```python
from build123d import *

# Parameters (mm, degrees)
SKETCH1_R           = 6.2992
BOSS_EXTRUDE1_DEPTH = 6.477
SKETCH2_R           = 9.4615
BOSS_EXTRUDE2_DEPTH = 6.223
SKETCH5_R           = 9.4615
SKETCH6_R           = 3.3782
SKETCH7_R           = 3.0226
CUT_EXTRUDE1_DEPTH  = 31.932950796


with BuildPart() as part:
    # Sketch1 → Boss-Extrude1 (new body)
    with BuildSketch(Plane(origin=(0, 0, 0), x_dir=(1, 0, 0), z_dir=(0, 1, 0))):
        with Locations(Location((0, 0, 0), (0, 0, 270))):
            Circle(SKETCH1_R)
    extrude(amount=BOSS_EXTRUDE1_DEPTH)

    # Sketch2 → Boss-Extrude2 (add)
    with BuildSketch(Plane(origin=(0, 6.477, 0), x_dir=(1, 0, 0), z_dir=(0, 1, 0))):
        with Locations(Location((0, 0, 0), (0, 0, 270))):
            Circle(SKETCH2_R)
    extrude(amount=BOSS_EXTRUDE2_DEPTH)

    # Sketch5 → Loft2 section 0
    with BuildSketch(Plane(origin=(0, 12.7, 0), x_dir=(1, 0, 0), z_dir=(0, 1, 0))):
        Circle(SKETCH5_R)
    # Sketch6 → Loft2 section 1
    with BuildSketch(Plane(origin=(0, 27.8892, 0), x_dir=(1, 0, 0), z_dir=(0, 1, 0))):
        Circle(SKETCH6_R)
    loft()

    # Sketch7 → Cut-Extrude1 (cut, through all)
    with BuildSketch(Plane(origin=(0, 27.8892, 0), x_dir=(1, 0, 0), z_dir=(0, 1, 0))):
        with Locations(Location((0, 0, 0), (0, 0, 270))):
            Circle(SKETCH7_R)
    extrude(amount=-CUT_EXTRUDE1_DEPTH, mode=Mode.SUBTRACT)


solid = part.part
```
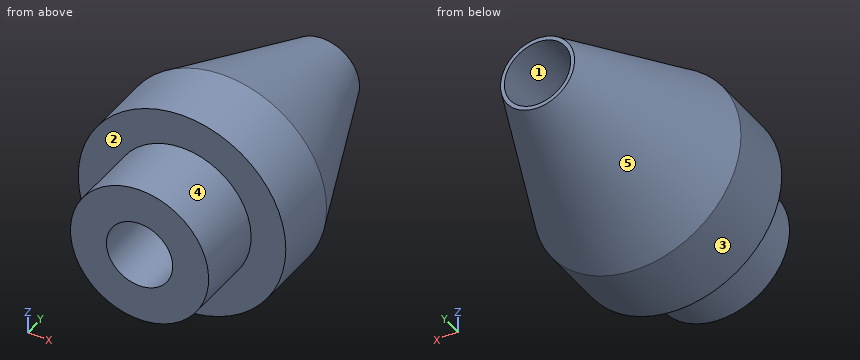
Check sheet for the modelled part. Datum: model origin and axes. Units: mm. Face numbers are marked on the shaded views. A direction names the side the tool comes from. Coordinates: 2 decimals unless noted, no trailing zeros. Write each loop counter-clockwise with the first axis right and the second up, starting at its lowest first coordinate (ties: lowest second). Pieces come first, ordered by that corner, then holes. Notation, with made-up numbers: (88, 37.5) -> (101, 37.5) arc R13 cw to (101, 61.5) -> close; hole circle Ø3 at (-9.5, -25). An arc over 180 degrees is marked (long way). Use a Markdown table: item, result.
1. Sectioned sample at A-A (x = 0). Enter the section's corners in (y, z).
Reported:
| item | result |
|---|---|
| outline | (0, -6.3) -> (6.48, -6.3) -> (6.48, -9.46) -> (12.7, -9.46) -> (27.89, -3.38) -> (27.89, -3.02) -> (0, -3.02) -> close; (0, 3.02) -> (27.89, 3.02) -> (27.89, 3.38) -> (12.7, 9.46) -> (6.48, 9.46) -> (6.48, 6.3) -> (0, 6.3) -> close |
2. Scan lines: line 1 along X through (y, z) = (6, 0); line 2 along X through (y, z) = (7.5, 0); line 3 along Z through (x, y) = (0.25, 10). Record each from-to range of solid material in increasing order.
Reported:
| item | result |
|---|---|
| line 1 | x = -6.3 to -3.02, 3.02 to 6.3 |
| line 2 | x = -9.46 to -3.02, 3.02 to 9.46 |
| line 3 | z = -9.46 to -3.01, 3.01 to 9.46 |
3. Sectioned sample at B-B (y = 11). Enter the section's corners in (x, z).
Reported:
| item | result |
|---|---|
| outline | circle Ø18.92 at (0, 0); hole circle Ø6.05 at (0, 0) |
4. Release check for a two-part mould opening along X. For the marked faces 1, 2 and 3 record: pulls with the +X half, pulls with the -X half, needs draft (parallel to the pull), parting line crosses it, or undercut.
Reported:
| item | result |
|---|---|
| face 1 | undercut |
| face 2 | needs draft |
| face 3 | parting line crosses it |
5. Go/stop test with flat-tipped pins: pin 1 Ø10 at (x, y) = (-5, 8.5) entering from +Z; pin 2 Ø3 at (x, y) = (5.5, 13.5) entering from +Z; pin 3 Ø10 at (x, y) = (-3.5, 17) entering from -Z; pin 4 Ø3 at (y, z) = (18.5, 2) entering from -X. Record where each tip stops, or that it passes through.
Reported:
| item | result |
|---|---|
| pin 1 | stops at z = 9.46 |
| pin 2 | stops at z = 8.46 |
| pin 3 | stops at z = -9.41 |
| pin 4 | stops at x = -7.56 |
6. Tool access check on the marked faces 4 and 5. Record the directions out of +Z, -Z, +X, -X, +Y, -Y that give a thin tool (end or side, any length) a straight path to the whole face; none if there is none.
Reported:
| item | result |
|---|---|
| face 4 | -Y |
| face 5 | +Y |
7. Sectioned sample at C-C (y = 3.25). Enter the section's corners in (x, z), plus the area to 3 significant figures.
Reported:
| item | result |
|---|---|
| outline | circle Ø12.6 at (0, 0); hole circle Ø6.05 at (0, 0) |
| area | 96.0 mm2 |
